```python
from build123d import *

# Parameters (mm, degrees)
ESBO_O1_W                 = 182
ESBO_O1_H                 = 10
CHANFRO1_SIZE             = 1
FURO_ROSCADO_DE_M61_D     = 5
FURO_ROSCADO_DE_M61_DEPTH = 17
FURO_ROSCADO_DE_M61_TIP   = 1.502151548
FURO_ROSCADO_DE_M62_D     = 5
FURO_ROSCADO_DE_M62_DEPTH = 17
FURO_ROSCADO_DE_M62_TIP   = 1.502151548


with BuildPart() as part:
    # Esboço1 → Revolução1 (revolve)
    with BuildSketch(Plane.XY, mode=Mode.PRIVATE) as revolu_o1_sk:
        with Locations((91, 5)):
            Rectangle(ESBO_O1_W, ESBO_O1_H)
    revolve(revolu_o1_sk.sketch.rotate(Axis((0, 0, 0), (1, 0, 0)), 90), axis=Axis((0, 0, 0), (1, 0, 0)))

    # Chanfro1
    chanfro1_edges = [part.edges().sort_by_distance(p)[0] for p in [
        (182, 0, -10),
        (0, 0, -10),
    ]]
    chamfer(chanfro1_edges, length=CHANFRO1_SIZE)

    # Furo roscado de M61
    with Locations(Plane(origin=(182, 0, 0), x_dir=(0, 0, -1), z_dir=(1, 0, 0))):
        with Locations((0, 0)):
            Hole(FURO_ROSCADO_DE_M61_D / 2, depth=FURO_ROSCADO_DE_M61_DEPTH)
            with Locations((0, 0, -(FURO_ROSCADO_DE_M61_DEPTH + FURO_ROSCADO_DE_M61_TIP / 2))):  # 118° drill point
                Cone(0, FURO_ROSCADO_DE_M61_D / 2, FURO_ROSCADO_DE_M61_TIP, mode=Mode.SUBTRACT)

    # Furo roscado de M62
    with Locations(Plane.ZY):
        with Locations((0, 0)):
            Hole(FURO_ROSCADO_DE_M62_D / 2, depth=FURO_ROSCADO_DE_M62_DEPTH)
            with Locations((0, 0, -(FURO_ROSCADO_DE_M62_DEPTH + FURO_ROSCADO_DE_M62_TIP / 2))):  # 118° drill point
                Cone(0, FURO_ROSCADO_DE_M62_D / 2, FURO_ROSCADO_DE_M62_TIP, mode=Mode.SUBTRACT)


solid = part.part
```
Design review of the part built by this model. Coordinates are the model's own, in mm. A direction names the side the tool comes from. Round coordinates to 2 decimals unless told otherwise and drop trailing zeros. Order: outer loops, then holes, each group sorted by start corner. A loop starts at its lowest first (then second) coordinate and runs counter-clockwise, first axis right, second up. Notation, with made-up numbers: M -10.5,77 L -0.5,77 A4 cw -0.5,81 Z; hole C -6.5,36 d5. An arc over 180 degrees is marked long. Put each result on its own line as item: value.
Q1. Consider section A-A (x = 132). State the section outline as (y, z) points.
Reported:
outline: C 0,0 d20
Q2. Insertion check: pin 1 Ø4 at (x, z) = (60, -5) entering from +Y; pin 2 Ø2 at (x, y) = (143.5, 2.5) entering from +Z; pin 3 Ø5 at (x, y) = (66.5, 4) entering from -Z. Each pin has a flat end and moves straight along its axis. Give the tip position at first contact, or say it passes through.
Reported:
pin 1: y = 9.54
pin 2: z = 9.89
pin 3: z = -9.89
Q3. Machinability: for faces 1 (the face through (0, 2, -2)), 2 (the face through (8.62, -2.44, 0.54)), 3 (the face through (173.38, -2.44, -0.54)), which of the approach directions +Z, -Z, +X, -X, +Y, -Y give a long, thin tool a straight path to every point of the face, cutting with its end or side? Answer none if there is none.
Reported:
face 1: +Z, -Z, -X, +Y, -Y
face 2: -X
face 3: +X
Q4. To check wall thickness, follow line 1 (Y direction, x = 174.5, z = 0); line 2 (Z direction, x = 156, y = -0.25); line 3 (Y direction, x = 7, z = -1.75). State the ranges of each line that lie inside material, in increasing order.
Reported:
line 1: -10 to -2.5, 2.5 to 10
line 2: -10 to 10
line 3: -9.85 to -1.79, 1.79 to 9.85
Q5. Draft analysis for pull direction Z (two halves, no side actions). For faces 4 (the face through (18.241, -0.424, -0.094)), 5 (the face through (92, 0, -10)), 6 (the face through (182, 2, -2)), state which applies: released by +Z, released by -Z, zero draft, split by the parting line, or undercut.
Reported:
face 4: undercut
face 5: split by the parting line
face 6: zero draft
